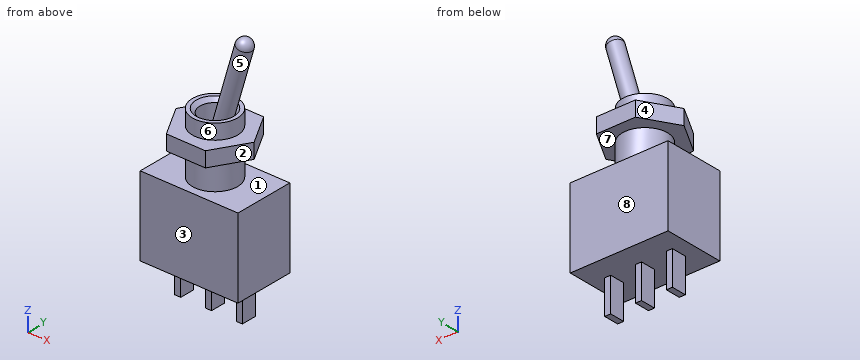
```python
from build123d import *

# Parameters (mm, degrees)
F1_DEPTH    = 4
F2_W        = 3
F2_H        = 4.5
F3_DEPTH    = 13.001
F4_R        = 3
F5_DEPTH    = 8
F8_DEPTH    = 2
F9_T        = 1
F9_T3_DEPTH = 2.8
F9_T5_DEPTH = 4
F9_T7_DEPTH = 2.8
F9_T9_DEPTH = 2.8
F11_SIZE    = 0.5
F13_R       = 1
F14_DEPTH   = 15
F15_R       = 1


# Not quite as in the source:
# - a shell that OpenCascade refuses in one call is made with other operations: the cavity is built on its own and cut out


with BuildPart() as f1:
    # F0 (on Front) → F1 (new body, symmetric)
    with BuildSketch(Plane.XZ):
        Polygon((6.5, -13.8051480774), (6.5, -3.3051480774), (-6.5, -3.3051480774), (-6.5, -13.8051480774), (-4.5, -13.8051480774), (-4.5, -18.3051480774), (-3.7, -18.3051480774), (-3.7, -13.8051480774), (-0.4, -13.8051480774), (-0.4, -18.3051480774), (0.4, -18.3051480774), (0.4, -13.8051480774), (3.7, -13.8051480774), (3.7, -18.3051480774), (4.5, -18.3051480774), (4.5, -13.8051480774), align=None)
    extrude(amount=F1_DEPTH, both=True)

    # F2 (on face) → F3 (cut, through all)
    with BuildSketch(Plane.YZ.offset(6.5)):
        with Locations((-2.5, -16.0551480774)):
            Rectangle(F2_W, F2_H)
        with Locations((2.5, -16.0551480774)):
            Rectangle(F2_W, F2_H)
    extrude(amount=-F3_DEPTH, mode=Mode.SUBTRACT)

    # F4 (on face) → F5 (join)
    with BuildSketch(Plane.XY.offset(-3.3051480774)):
        Circle(F4_R)
    extrude(amount=F5_DEPTH)

    # F7 (on offset) → F8 (join)
    with BuildSketch(Plane.XY.offset(0.6948519226)):
        Polygon((2.5980762114, -4.5), (5.1961524227, 0), (2.5980762114, 4.5), (-2.5980762114, 4.5), (-5.1961524227, 0), (-2.5980762114, -4.5), align=None)
    extrude(amount=F8_DEPTH)

    # F9: shell of thickness 1, made by hand


with BuildPart() as f9_core1:
    # F9_t2: copy of F1
    add(f1.part)

    # the walls: a layer under each face that stays
    f9_faces = [f9_core1.faces().sort_by_distance(p)[0] for p in [
        (-4.3333333333, 2.6666666667, -13.8051480774),
        (6.5, 0, -8.5551480774),
        (0, -4, -8.5551480774),
        (-6.5, 0, -8.5551480774),
        (0, 4, -8.5551480774),
        (0, 1, -16.0551480774),
        (-0.4, 0, -16.0551480774),
        (0, -1, -16.0551480774),
        (0.4, 0, -16.0551480774),
        (3.7, 0, -16.0551480774),
        (4.1, -1, -16.0551480774),
        (4.5, 0, -16.0551480774),
        (4.1, 1, -16.0551480774),
        (-4.1, 1, -16.0551480774),
        (-4.5, 0, -16.0551480774),
        (-4.1, -1, -16.0551480774),
        (-3.7, 0, -16.0551480774),
        (4.3333333333, 2.6666666667, -3.3051480774),
        (0, 0, -18.3051480774),
        (4.1, 0, -18.3051480774),
        (-4.1, 0, -18.3051480774),
        (-3, 0, -1.3051480774),
        (-3.4641016151, 0, 0.6948519226),
        (-3.897114317, -2.25, 1.6948519226),
        (-3.897114317, 2.25, 1.6948519226),
        (0, -4.5, 1.6948519226),
        (0, 4.5, 1.6948519226),
        (3.897114317, -2.25, 1.6948519226),
        (3.897114317, 2.25, 1.6948519226),
        (-3.4641016151, 0, 2.6948519226),
        (-3, 0, 3.6948519226),
    ]]
    thicken(f9_faces, amount=-F9_T, mode=Mode.SUBTRACT)

    # F9_s4 → F9_t3 (cut)
    with BuildSketch(Plane.YZ.offset(-1.4)):
        Polygon((1.01, -13.8151480774), (1, -12.8051480774), (0, -12.8051480774), (0, -13.8051480774), align=None)
        Polygon((-1.01, -13.8151480774), (-1, -12.8051480774), (0, -12.8051480774), (0, -13.8051480774), align=None)
    extrude(amount=F9_T3_DEPTH, mode=Mode.SUBTRACT)

    # F9_s6 → F9_t5 (cut)
    with BuildSketch(Plane.XZ.offset(-2)):
        Polygon((-0.41, -13.8151480774), (-0.4, -12.8051480774), (0.6, -12.8051480774), (0.6, -13.8051480774), align=None)
        Polygon((0.41, -13.8151480774), (0.4, -12.8051480774), (-0.6, -12.8051480774), (-0.6, -13.8051480774), align=None)
        Polygon((3.69, -13.8151480774), (3.7, -12.8051480774), (4.7, -12.8051480774), (4.7, -13.8051480774), align=None)
        Polygon((4.51, -13.8151480774), (4.5, -12.8051480774), (3.5, -12.8051480774), (3.5, -13.8051480774), align=None)
        Polygon((-4.51, -13.8151480774), (-4.5, -12.8051480774), (-3.5, -12.8051480774), (-3.5, -13.8051480774), align=None)
        Polygon((-3.69, -13.8151480774), (-3.7, -12.8051480774), (-4.7, -12.8051480774), (-4.7, -13.8051480774), align=None)
    extrude(amount=F9_T5_DEPTH, mode=Mode.SUBTRACT)

    # F9_s8 → F9_t7 (cut)
    with BuildSketch(Plane.YZ.offset(2.7)):
        Polygon((-1.01, -13.8151480774), (-1, -12.8051480774), (0, -12.8051480774), (0, -13.8051480774), align=None)
        Polygon((1.01, -13.8151480774), (1, -12.8051480774), (0, -12.8051480774), (0, -13.8051480774), align=None)
    extrude(amount=F9_T7_DEPTH, mode=Mode.SUBTRACT)

    # F9_s10 → F9_t9 (cut)
    with BuildSketch(Plane.YZ.offset(-5.5)):
        Polygon((1.01, -13.8151480774), (1, -12.8051480774), (0, -12.8051480774), (0, -13.8051480774), align=None)
        Polygon((-1.01, -13.8151480774), (-1, -12.8051480774), (0, -12.8051480774), (0, -13.8051480774), align=None)
    extrude(amount=F9_T9_DEPTH, mode=Mode.SUBTRACT)

    # F9_s11 → F9_t12 (revolve, cut)
    with BuildSketch(Plane.XZ):
        Polygon((3.01, -3.2951480774), (3, -4.3051480774), (2, -4.3051480774), (2, -3.3051480774), align=None)
    revolve(axis=Axis((0, 0, -3.3051480774), (0, 0, 1)), mode=Mode.SUBTRACT)

    # F9_s13 → F9_t14 (revolve, cut)
    with BuildSketch(Plane.XZ):
        Polygon((3.01, 0.6848519226), (2, 0.6948519226), (2, 1.6948519226), (3, 1.6948519226), align=None)
    revolve(axis=Axis((0, 0, 0.6948519226), (0, 0, -1)), mode=Mode.SUBTRACT)

    # F9_s15 → F9_t16 (revolve, cut)
    with BuildSketch(Plane.XZ):
        Polygon((3.01, 2.7048519226), (3, 1.6948519226), (2, 1.6948519226), (2, 2.6948519226), align=None)
    revolve(axis=Axis((0, 0, 2.6948519226), (0, 0, -1)), mode=Mode.SUBTRACT)


with BuildPart() as f1_1:
    add(f1.part)

    # what is left inside the walls is the cavity
    f9_cavity = [f9_core1.part.solids().sort_by_distance(p)[0] for p in [
        (0, 2.99, -9.971815),
    ]]
    add(f9_cavity, mode=Mode.SUBTRACT)

    # F11
    f11_edges = [f1_1.edges().sort_by_distance(p)[0] for p in [
        (-2, 0, 4.694852),
    ]]
    chamfer(f11_edges, length=F11_SIZE)

    # F13 (on line) → F14 (join)
    with BuildSketch(Plane(origin=(0, 0, 0), x_dir=(0.9597844806, 0, -0.2807378684), z_dir=(0.2807378684, 0, 0.9597844806))):
        Circle(F13_R)
    extrude(amount=F14_DEPTH)

    # F15
    f15_edges = [f1_1.edges().sort_by_distance(p)[0] for p in [
        (3.251284, 0, 14.677505),
    ]]
    fillet(f15_edges, radius=F15_R)


solid = f1_1.part
```
Geometry check sheet. Reference: the model listing, model coordinates, mm. Face numbers are marked on the shaded views. A direction names the side the tool comes from. Round coordinates to 2 decimals unless told otherwise and drop trailing zeros. Loops run counter-clockwise (first coordinate to the right, second up) from the corner with the lowest first, then second, coordinate; pieces in that order, holes last. Notation, with made-up numbers: (9.25, -0.5) - (63.25, -0.5) arc R31 ccw to (63.25, 29.5) - close; hole circle Ø10 at (-9, 12). An arc over 180 degrees is marked (long way). Write each question's results on one line, items separated by ' | '. Start each with the question number.
Q1. Cross-section at B-B on x = -4. Enter the section's corners in (y, z).
Q2. Release check for a two-part mould opening along Y. For the marked faces 5, 6, 7 and 8 record: +Y half, -Y half, draft (parallel to the pull), parting line (faces both ways), or undercut.
Q3. Gauge pin test, flat ends, axial feed: P1, Ø0.6, axis at x = 4, z = -16, coming from the -Y side; P2, Ø1.6, axis at y = 0, z = -15.5, coming from the +X side; P3, Ø1.5, axis at y = -2.5, z = -3, coming from the +X side; P4, Ø2.5, axis at x = -2, z = -10.5, coming from the +Y side. Record the tip position at first contact, or that the pin passes through.
Q4. Thickness scan on line 1 (X direction, y = 1.5, z = -10); line 2 (Y direction, x = 0, z = -2.25); line 3 (Z direction, x = 0.75, y = 3.25). Record the ranges inside material, lowest first. Write a range as [from, to].
Q5. Cross-section at A-A on z = -11.5. Enter the section's corners in (x, y).
Q6. Access from +Z, -Z, +X, -X, +Y, -Y to the whole of each face (thin tool, end or side, straight path). Record for the marked faces 1, 2, 3 and 4.
Answers below:
1) outline: (-4, -13.81) - (-1, -13.81) - (-1, -18.31) - (1, -18.31) - (1, -13.81) - (4, -13.81) - (4, -3.31) - (-4, -3.31) - close; (-2.07, 0.69) - (2.07, 0.69) - (2.07, 2.69) - (-2.07, 2.69) - close; hole (-3, -12.81) - (3, -12.81) - (3, -4.31) - (-3, -4.31) - close
2) face 5: undercut | face 6: parting line | face 7: draft | face 8: +Y half
3) P1: stops at y = -1 | P2: stops at x = 4.5 | P3: stops at x = 6.5 | P4: stops at y = 4
4) line 1: x = [-6.5, -5.5], [5.5, 6.5] | line 2: y = [-3, -2], [2, 3] | line 3: z = [-13.81, -3.31], [0.69, 2.69]
5) outline: (-6.5, -4) - (6.5, -4) - (6.5, 4) - (-6.5, 4) - close; hole (-5.5, -3) - (5.5, -3) - (5.5, 3) - (-5.5, 3) - close
6) face 1: none | face 2: +Z, +X, -Y | face 3: -Z, +X, -X, -Y | face 4: +Z, -X, +Y
